Work out the finished part from the listing and answer in its coordinate system (mm). A direction names the side the tool comes from. Coordinates: 2 decimals unless noted, no trailing zeros. Order: outer loops, then holes, each group sorted by start corner. A loop starts at its lowest first (then second) coordinate and runs counter-clockwise, first axis right, second up.
1. The part is cut by section B-B, the plane z = 2.75. Give the vertices of the cut face in (x, y) (3 decimals), then the cut area to 3 significant figures.
2. The part is cut by section A-A, the plane x = 0. Give the vertices of the cut face in (y, z) (3 decimals).
3. A tool of negligible diameter and unlimited length cuts with its end or side. For faces 5 (the flat face through (-10, -12, 4)), 6 (the flat face through (0, 18, 7)), 7 (the flat face through (16, -1, 4.5)), 8 (the flat face through (15, -8, 4)), from which of +Z, -Z, +X, -X, +Y, -Y can it reach the whole face along a straight path? Write none if from no direction.
4. Flat-ended cylindrical pins translate along their axes: pin 1 Ø6.5 at (x, y) = (14, 1) entering from +Z; pin 2 Ø3.5 at (x, y) = (12.5, 40) entering from +Z; pin 3 Ø2.5 at (x, y) = (0, 0) entering from -Z; pin 4 Ø0.6 at (y, z) = (-11.5, 4.5) entering from +X. Find the tip coordinate at first contact, or state that the pin passes through.
5. The part is cut by section D-D, the plane x = -14. Give the vertices of the cut face in (y, z).
6. The part is cut by section C-C, the plane y = 30. Give the vertices of the cut face in (x, z).
7. Find the intervals of material crossed by probe 1 along Y at (x, z) = (-14, 2); probe 2 along Y at (x, z) = (0, 4.25) (3 decimals); probe 3 along Y at (x, z) = (-14, 5.45), in increasing order.
8. Determine the mould class of faces 1 (the flat face through (0, 50, 3)), 2 (the cylindrical face through (9.248, -14.287, 4.056)), 3 (the cylindrical face through (-1.24, 39.42, 3.55)), 4 (the flat face through (0, 18, 0)) for opening direction Y: +Y half, -Y half, draft (parallel to the pull), parting line (faces both ways), or undercut.
```python
from build123d import *
from build123d.topology import SkipClean

# Parameters (mm, degrees)
SKETCH1_R           = 2.125
BOSS_EXTRUDE2_DEPTH = 8
SKETCH7_W           = 40
SKETCH7_H           = 58
BOSS_EXTRUDE3_DEPTH = 8
FILLET1_R           = 2.5
SKETCH3_R           = 9.5
CUT_EXTRUDE2_DEPTH  = 55.442630355
SKETCH2_R           = 2.05
CUT_EXTRUDE1_DEPTH  = 55.442630355
SKETCH6_W           = 60
SKETCH6_H           = 50
CUT_EXTRUDE5_DEPTH  = 1
SKETCH9_R           = 2.125
CUT_EXTRUDE7_DEPTH  = 55.442630355
SKETCH11_R          = 3.5
CUT_EXTRUDE9_DEPTH  = 3.5


with BuildPart() as part:
    # Sketch1 → Boss-Extrude2 (new body)
    with BuildSketch(Plane.XY):
        with BuildLine():
            Line((-10, -15), (-10, 15))
            Line((-10, 15), (-15, 30))
            ThreePointArc((-15, 30), (0, 45), (15, 30))
            Line((15, 30), (10, 15))
            Line((10, 15), (10, -15))
            Line((10, -15), (-10, -15))
        make_face()
        Circle(SKETCH1_R, mode=Mode.SUBTRACT)
        with Locations((0, -10)):
            Circle(SKETCH1_R, mode=Mode.SUBTRACT)
    extrude(amount=BOSS_EXTRUDE2_DEPTH)

    # Sketch7 → Boss-Extrude3 (add)
    with BuildSketch(Plane(origin=(0, 0, 0), x_dir=(-1, 0, 0), z_dir=(0, 0, -1))):
        with Locations((0, 21)):
            Rectangle(SKETCH7_W, SKETCH7_H)
    extrude(amount=-BOSS_EXTRUDE3_DEPTH)

    # Fillet1
    fillet1_edges = [part.edges().sort_by_distance(p)[0] for p in [
        (10, -15, 4),
        (-10, -15, 4),
        (-20, -8, 4),
        (-10, -8, 4),
        (10, -8, 4),
        (-20, 50, 4),
        (20, 50, 4),
        (20, -8, 4),
    ]]
    fillet(fillet1_edges, radius=FILLET1_R)

    # Sketch3 → Cut-Extrude2 (cut, through all)
    with BuildSketch(Plane.XY.offset(8)):
        with Locations((0, 30)):
            Circle(SKETCH3_R)
    extrude(amount=-CUT_EXTRUDE2_DEPTH, mode=Mode.SUBTRACT)

    # Sketch2 → Cut-Extrude1 (cut, through all)
    with BuildSketch(Plane.XY.offset(8)):
        with Locations((-14, 41)):
            Circle(SKETCH2_R)
        with Locations((14, 41)):
            Circle(SKETCH2_R)
        with Locations((14, 1)):
            Circle(SKETCH2_R)
        with Locations((-14, 1)):
            Circle(SKETCH2_R)
    extrude(amount=-CUT_EXTRUDE1_DEPTH, mode=Mode.SUBTRACT)

    # Sketch6 → Cut-Extrude5 (cut)
    with BuildSketch(Plane.XY.offset(8)):
        with Locations((0, 30)):
            Rectangle(SKETCH6_W, SKETCH6_H)
    extrude(amount=-CUT_EXTRUDE5_DEPTH, mode=Mode.SUBTRACT)

    # Sketch9 → Cut-Extrude7 (cut, through all)
    with SkipClean():  # the faces are left unmerged after this step: merging them gives an invalid solid
        with BuildSketch(Plane.XY.offset(8)):
            with Locations((0, -10)):
                Circle(SKETCH9_R)
            Circle(SKETCH9_R)
        extrude(amount=-CUT_EXTRUDE7_DEPTH, mode=Mode.SUBTRACT)

    # Sketch11 → Cut-Extrude9 (cut)
    with SkipClean():  # the faces are left unmerged after this step: merging them gives an invalid solid
        with BuildSketch(Plane.XY.offset(8)):
            with Locations((-14, 1)):
                Circle(SKETCH11_R)
            with Locations((14, 1)):
                Circle(SKETCH11_R)
            with Locations((14, 41)):
                Circle(SKETCH11_R)
            with Locations((-14, 41)):
                Circle(SKETCH11_R)
        extrude(amount=-CUT_EXTRUDE9_DEPTH, mode=Mode.SUBTRACT)


solid = part.part
```
Geometry says:
1. outline: (-20, -5.5) arc R2.5 ccw to (-17.5, -8) - (-12.5, -8) arc R2.5 cw to (-10, -10.5) - (-10, -12.5) arc R2.5 ccw to (-7.5, -15) - (7.5, -15) arc R2.5 ccw to (10, -12.5) - (10, -10.5) arc R2.5 cw to (12.5, -8) - (17.5, -8) arc R2.5 ccw to (20, -5.5) - (20, 47.5) arc R2.5 ccw to (17.5, 50) - (-17.5, 50) arc R2.5 ccw to (-20, 47.5) - close; hole circle Ø4.1 at (-14, 1); hole circle Ø4.1 at (-14, 41); hole circle Ø19 at (0, 30); hole circle Ø4.25 at (0, -10); hole circle Ø4.25 at (0, 0); hole circle Ø4.1 at (14, 1); hole circle Ø4.1 at (14, 41)
1. area: 2,090 mm2
2. outline: (-15, 0) - (-12.125, 0) - (-12.125, 8) - (-15, 8) - close; (-7.875, 0) - (-2.125, 0) - (-2.125, 8) - (-7.875, 8) - close; (2.125, 0) - (20.5, 0) - (20.5, 7) - (5, 7) - (5, 8) - (2.125, 8) - close; (39.5, 0) - (50, 0) - (50, 7) - (39.5, 7) - close
3. face 5: +Z, -Z, -X, -Y
3. face 6: +Z, +X, -X, +Y
3. face 7: +Z
3. face 8: +Z, -Z, +X, -Y
4. pin 1: stops at z = 4.5
4. pin 2: stops at z = 7
4. pin 3: passes through
4. pin 4: stops at x = 10
5. outline: (-8, 0) - (-1.05, 0) - (-1.05, 4.5) - (-2.5, 4.5) - (-2.5, 8) - (-8, 8) - close; (3.05, 0) - (38.95, 0) - (38.95, 4.5) - (37.5, 4.5) - (37.5, 7) - (5, 7) - (5, 8) - (4.5, 8) - (4.5, 4.5) - (3.05, 4.5) - close; (43.05, 0) - (50, 0) - (50, 7) - (44.5, 7) - (44.5, 4.5) - (43.05, 4.5) - close
6. outline: (-20, 0) - (-9.5, 0) - (-9.5, 7) - (-20, 7) - close; (9.5, 0) - (20, 0) - (20, 7) - (9.5, 7) - close
7. probe 1: y = -8 to -1.05, 3.05 to 38.95, 43.05 to 50
7. probe 2: y = -15 to -12.125, -7.875 to -2.125, 2.125 to 20.5, 39.5 to 50
7. probe 3: y = -8 to -2.5, 4.5 to 37.5, 44.5 to 50
8. face 1: +Y half
8. face 2: -Y half
8. face 3: undercut
8. face 4: draft
